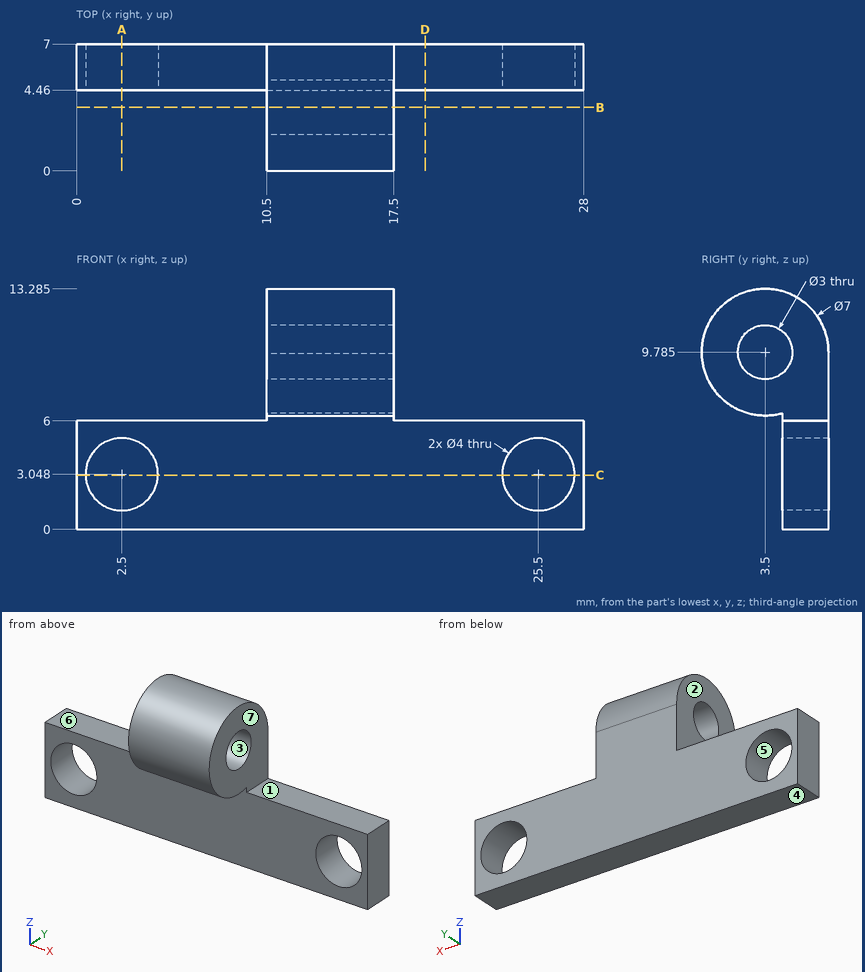
For this review, use the dimensioned drawing (mm, ordinates from the lowest corner) and the shaded views. A direction names the side the tool comes from. Round coordinates to 2 decimals unless told otherwise and drop trailing zeros. Write each loop counter-clockwise with the first axis right and the second up, starting at its lowest first coordinate (ties: lowest second). Pieces come first, ordered by that corner, then holes. Notation, with made-up numbers: (82, 29.5) - (114, 29.5) arc R26 cw to (114, 58.5) - close; hole circle Ø4 at (37, 10.5). An arc over 180 degrees is marked (long way). Use a Markdown table: item, result.
Q1. The part is to be moulded in two halves that separate along Z. For the marked faces 4, 5, 6 and 7, say which applies: pulls with the +Z half, pulls with the -Z half, needs draft (parallel to the pull), parting line crosses it, or undercut.
Derived:
| item | result |
|---|---|
| face 4 | pulls with the -Z half |
| face 5 | undercut |
| face 6 | pulls with the +Z half |
| face 7 | needs draft |
Q2. We need section C-C (z = 3). Give the boundary of the cut face in (x, y), plus the area to 3 significant figures.
Derived:
| item | result |
|---|---|
| outline | (0, 4.46) - (0.5, 4.46) - (0.5, 7) - (0, 7) - close; (4.5, 4.46) - (23.5, 4.46) - (23.5, 7) - (4.5, 7) - close; (27.5, 4.46) - (28, 4.46) - (28, 7) - (27.5, 7) - close |
| area | 50.8 mm2 |
Q3. We need section D-D (x = 19.25). Give the boundary of the cut face in (y, z).
Derived:
| item | result |
|---|---|
| outline | (4.46, 0) - (7, 0) - (7, 6) - (4.46, 6) - close |
Q4. We need section B-B (y = 3.5). Give the boundary of the cut face in (x, z) (1 decimal), plus the area to 3 significant figures.
Derived:
| item | result |
|---|---|
| outline | (10.5, 6.3) - (17.5, 6.3) - (17.5, 8.3) - (10.5, 8.3) - close; (10.5, 11.3) - (17.5, 11.3) - (17.5, 13.3) - (10.5, 13.3) - close |
| area | 28.0 mm2 |
Q5. Machinability: for the marked faces 1, 2 and 3, which of the approach directions +Z, -Z, +X, -X, +Y, -Y give a long, thin tool a straight path to every point of the face, cutting with its end or side? Answer none if there is none.
Derived:
| item | result |
|---|---|
| face 1 | +Z, +X, +Y, -Y |
| face 2 | +Z, -X, +Y, -Y |
| face 3 | +X, -X |
Q6. Clearance check with flat-ended pins moving along their axes: pin 1 (2.5 mm diameter, centred on x = 2.5, z = 3.048, fed in from +Y); pin 2 (5 mm diameter, centred on x = 18, z = 4.5, fed in from -Y); pin 3 (0.8 mm diameter, centred on x = 24.5, y = 6.5, fed in from +Z); pin 4 (3.5 mm diameter, centred on y = 2, z = 9.5, fed in from -X). State where each tip first meets the part, or that it passes through.
Derived:
| item | result |
|---|---|
| pin 1 | passes through |
| pin 2 | stops at y = 1.45 |
| pin 3 | stops at z = 6 |
| pin 4 | stops at x = 10.5 |
Q7. We need section A-A (x = 2.5). Give the boundary of the cut face in (y, z).
Derived:
| item | result |
|---|---|
| outline | (4.46, 0) - (7, 0) - (7, 1.05) - (4.46, 1.05) - close; (4.46, 5.05) - (7, 5.05) - (7, 6) - (4.46, 6) - close |
Q8. Wall thickness on line 1 along Z through (x, y) = (2.5, 5.2); line 2 along X through (y, z) = (5.25, 2.75); line 3 along X through (y, z) = (4.5, 3.5): over which ranges is each line inside the solid? List them lowest first.
Derived:
| item | result |
|---|---|
| line 1 | z = 0 to 1.05, 5.05 to 6 |
| line 2 | x = 0 to 0.52, 4.48 to 23.52, 27.48 to 28 |
| line 3 | x = 0 to 0.55, 4.45 to 23.55, 27.45 to 28 |
